Here's how the part is built. I have some questions about the finished solid (model axes, mm). A direction names the side the tool comes from. Give positions to 0.01 mm unless a question says otherwise; leave off trailing zeros. Loops run counter-clockwise (first coordinate to the right, second up) from the corner with the lowest first, then second, coordinate; pieces in that order, holes last. Notation, with made-up numbers: (52, 6.25) - (90, 6.25) arc R30 ccw to (90, 44.25) - close; hole circle Ø6 at (56.5, 50.25). An arc over 180 degrees is marked (long way). Return JSON: item names as keys, results as strings. Group by question number.
(1) If we section it at C-C (z = -113): Please give me the cut outline in (x, y).
(2) If we section it at B-B (y = -4.75): State how many separate pieces and enclosed holes the cut face has, then the cut area to 3 significant figures.
(3) If we mould it in two halves opening along X, with no side actions, what happens to faces 1 (the flat face through (0, -6, 0)), 2 (the cylindrical face through (-3.26, -8.39, -104.56)), 3 (the flat face through (0, -3, -5.382))? For each: released by +X, released by -X, zero draft, split by the parting line, or undercut.
(4) If we section it at D-D (y = -11.5): Please give me the cut outline in (x, z), then the cut area to 3 significant figures.
(5) I need wall thicknesses on probe 1 along Y at (x, z) = (-0.5, -85.5); probe 2 along Z at (x, y) = (-10.75, -4.5); probe 3 along Z at (x, y) = (12.5, -6.5). Which ranges of each line are inside material? Lowest first, please. Write a range as [from, to].
(6) On a 3-axis mill with a long thin cutter (end or side, diameter ignored), from which of +Z, -Z, +X, -X, +Y, -Y can I reach the whole of each face in a straight line? I mean faces 4 (the flat face through (-3.707, -1.479, -144.708)), 5 (the flat face through (0, -1, -159)), 6 (the conical face through (-0.131, -5.957, -154.647)), 7 (the flat face through (-3, -6, -100)). Say none if no direction works.
(7) If we section it at A-A (z = -24): Please give me the cut outline in (x, y), then the cut area to 3 significant figures.
(8) For P1, Ø2, axis at y = -9, z = -37.5, coming from the -X side; P2, Ø2.5, axis at y = -1.5, z = -103.5, coming from the -X side; P3, Ø3, axis at x = -2, z = -23.5, coming from the +Y side, each with a flat end and sliding along its axis, tell me the tip position at first contact or that it passes through.
```python
from build123d import *

# Parameters (mm, degrees)
REVOLVE1_ANGLE          = 180
SKETCH3_W               = 24.5
SKETCH3_H               = 53.5
CUT_EXTRUDE1_DEPTH      = 7
CUT_EXTRUDE2_DEPTH      = 3
SKETCH5_W               = 2.5
SKETCH5_H               = 3.617532458
CUT_EXTRUDE3_DEPTH      = 3
CUT_EXTRUDE4_REACH      = 168.114
CUT_EXTRUDE4_END_RADIUS = 9
SKETCH6_W               = 6
SKETCH6_H               = 10
SKETCH7_W               = 4.455882352
SKETCH7_H               = 15
CUT_EXTRUDE5_DEPTH      = 1
SKETCH8_W               = 5
SKETCH8_H               = 3.617532458
CUT_EXTRUDE6_DEPTH      = 3
CHAMFER10_SIZE          = 2
CHAMFER10_SIZE_2        = 3.464101615
FILLET1_R               = 3


with BuildPart() as part:
    # Sketch2 → Revolve1 (revolve)
    with BuildSketch(Plane(origin=(0, 0, 0), x_dir=(1, 0, 0), z_dir=(0, 1, 0))):
        Polygon((0, 0), (-15, 0), (-15, 64), (-9, 64), (-9, 144), (-3, 165), (0, 165), align=None)
    revolve(axis=Axis((0, 0, -165), (0, 0, 1)), revolution_arc=REVOLVE1_ANGLE)

    # Sketch3 → Cut-Extrude1 (cut)
    with BuildSketch(Plane(origin=(0, 0, 0), x_dir=(1, 0, 0), z_dir=(0, 1, 0))):
        with Locations((0, 32.132467542)):
            Rectangle(SKETCH3_W, SKETCH3_H)
    extrude(amount=-CUT_EXTRUDE1_DEPTH, mode=Mode.SUBTRACT)

    # Sketch4 → Cut-Extrude2 (cut)
    with BuildSketch(Plane(origin=(0, 0, 0), x_dir=(1, 0, 0), z_dir=(0, 1, 0))):
        Polygon((-6, 62.5), (6, 62.5), (6, 136.5), (1.25, 153.5), (-1.25, 153.5), (-6, 136.5), align=None)
    extrude(amount=-CUT_EXTRUDE2_DEPTH, mode=Mode.SUBTRACT)

    # Sketch5 → Cut-Extrude3 (cut)
    with BuildSketch(Plane(origin=(0, 0, 0), x_dir=(1, 0, 0), z_dir=(0, 1, 0))):
        with Locations((-3.75, 60.691233771)):
            Rectangle(SKETCH5_W, SKETCH5_H)
        with Locations((3.75, 60.691233771)):
            Rectangle(SKETCH5_W, SKETCH5_H)
    extrude(amount=-CUT_EXTRUDE3_DEPTH, mode=Mode.SUBTRACT)

    # Cut-Extrude4: up to this cylinder (the profile starts inside it)
    cut_extrude4_end = Plane(origin=(0, 0, -100.5), z_dir=(0, 0, -1)) * Cylinder(CUT_EXTRUDE4_END_RADIUS, 355.228, mode=Mode.PRIVATE)
    # Sketch6 → Cut-Extrude4 (cut, up to the surface)
    with BuildSketch(Plane(origin=(0, -3, 0), x_dir=(1, 0, 0), z_dir=(0, 1, 0)), mode=Mode.PRIVATE) as cut_extrude4_sk1:
        with Locations((0, 100.5)):
            Rectangle(SKETCH6_W, SKETCH6_H)
    cut_extrude4_tool1 = extrude(cut_extrude4_sk1.sketch, amount=-CUT_EXTRUDE4_REACH, mode=Mode.PRIVATE) & cut_extrude4_end
    add(cut_extrude4_tool1.solids().sort_by_distance((0, -3, -100.5))[0], mode=Mode.SUBTRACT)

    # Sketch7 → Cut-Extrude5 (cut)
    with BuildSketch(Plane(origin=(0, 0, 0), x_dir=(1, 0, 0), z_dir=(0, 1, 0))):
        with Locations((0, 157.5)):
            Rectangle(SKETCH7_W, SKETCH7_H)
    extrude(amount=-CUT_EXTRUDE5_DEPTH, mode=Mode.SUBTRACT)

    # Sketch8 → Cut-Extrude6 (cut)
    with BuildSketch(Plane(origin=(0, 0, 0), x_dir=(1, 0, 0), z_dir=(0, 1, 0))):
        with Locations((0, 60.691233771)):
            Rectangle(SKETCH8_W, SKETCH8_H)
    extrude(amount=-CUT_EXTRUDE6_DEPTH, mode=Mode.SUBTRACT)

    # Chamfer10
    # the kernel refuses this chamfer: 3.464101615, 2 mm, written as the material it takes off along each edge
    with BuildSketch(Plane(origin=(10.211927941, -1, -153.5), x_dir=(0, 0.05789386240267106, -0.9983227437537926), z_dir=(-1, 0, 0))) as chamfer10_piece_1_section:
        Polygon((CHAMFER10_SIZE * 0.998322743754, CHAMFER10_SIZE * 0.0578938624027), (-CHAMFER10_SIZE_2 * 0.057893862405, CHAMFER10_SIZE_2 * 0.998322743793), (0, 0), align=None)
    chamfer10_piece_1 = extrude(amount=20.423855882, mode=Mode.PRIVATE)
    chamfer10_piece_1 = split(chamfer10_piece_1, bisect_by=Plane(origin=(0, -3, -154.190565485), z_dir=(0, 1, 0)), keep=Keep.TOP, mode=Mode.PRIVATE)
    chamfer10_piece_1 = split(chamfer10_piece_1, bisect_by=Plane(origin=(-0.980499377, -1.889149357, -154.464528546), z_dir=(0.9631109740028581, 6.725367985932025e-15, 0.26910453685374025)), keep=Keep.TOP, mode=Mode.PRIVATE)
    chamfer10_piece_1 = split(chamfer10_piece_1, bisect_by=Plane(origin=(0.980499377, -1.889149357, -154.464528546), z_dir=(-0.9631109740028581, -6.725367985932025e-15, 0.26910453685374025)), keep=Keep.TOP, mode=Mode.PRIVATE)
    add(chamfer10_piece_1, mode=Mode.SUBTRACT)

    # Fillet1
    fillet1_edges = [part.edges().sort_by_distance(p)[0] for p in [
        (0, -1, -155.5),
    ]]
    fillet(fillet1_edges, radius=FILLET1_R)


solid = part.part
```
Values:
{
 "1": {"outline": "(-9, 0) arc R9 ccw to (9, 0) - (6, 0) - (6, -3) - (-6, -3) - (-6, 0) - close"},
 "2": {"separate pieces": "1", "enclosed holes": "2", "area": "1,820 mm2"},
 "3": {"face 1": "zero draft", "face 2": "split by the parting line", "face 3": "undercut"},
 "4": {"outline": "(-9.63, -64) - (9.63, -64) - (9.63, 0) - (-9.63, 0) - close", "area": "1,230 mm2"},
 "5": {"probe 1": "[-8.99, -3]", "probe 2": "[-64, -58.88], [-5.38, 0]", "probe 3": "[-64, 0]"},
 "6": {"face 4": "+Y", "face 5": "-Z, +Y", "face 6": "-Z, -Y", "face 7": "+Y, -Y"},
 "7": {"outline": "(-15, 0) arc R15 ccw to (15, 0) - (12.25, 0) - (12.25, -7) - (-12.25, -7) - (-12.25, 0) - close", "area": "182 mm2"},
 "8": {"P1": "x = -12.69", "P2": "x = -9", "P3": "y = -7"}
}
